Check sheet for the modelled part. Datum: model origin and axes. Units: mm. Face numbers are marked on the shaded views. A direction names the side the tool comes from. Round coordinates to 2 decimals unless told otherwise and drop trailing zeros. Write each loop counter-clockwise with the first axis right and the second up, starting at its lowest first coordinate (ties: lowest second). Pieces come first, ordered by that corner, then holes. Notation, with made-up numbers: (-34, 85) -> (7, 85) arc R24 cw to (7, 105) -> close; hole circle Ø8 at (67, -0.5). An arc over 180 degrees is marked (long way). One line per item, written item: value.
from build123d import *

# Parameters (mm, degrees)
SKETCH1_R           = 33.5
SKETCH1_R_2         = 30
BOSS_EXTRUDE1_DEPTH = 76.5
SKETCH3_R           = 33.5
BOSS_EXTRUDE2_DEPTH = 16.5
SKETCH4_W           = 20
SKETCH4_H           = 3.5
BOSS_EXTRUDE4_DEPTH = 30.867
SKETCH4_5_W         = 11
SKETCH4_5_H         = 3.5
BOSS_EXTRUDE5_DEPTH = 27
SKETCH4_7_R         = 1.25
CUT_EXTRUDE1_DEPTH  = 90.981942633
FILLET1_R           = 3.5
FILLET2_R           = 1.5
CUT_EXTRUDE4_DEPTH  = 103.136868955
BOSS_EXTRUDE7_START = 3
SKETCH6_10_R        = 10
BOSS_EXTRUDE7_DEPTH = 3
SKETCH12_R          = 5
SKETCH12_R_2        = 3
BOSS_EXTRUDE8_DEPTH = 1.5
SKETCH12_3_R        = 1.5
CUT_EXTRUDE7_DEPTH  = 101.439733174
CIRPATTERN1_COUNT   = 4
SKETCH12_4_R        = 1.5
CUT_EXTRUDE8_DEPTH  = 101.439733174
CUT_EXTRUDE9_DEPTH  = 90.981942633
CIRPATTERN2_COUNT   = 4
SKETCH13_W          = 60
SKETCH13_H          = 27
CUT_EXTRUDE11_DEPTH = 33.5
BOSS_EXTRUDE9_START = -3.5
SKETCH14_R          = 33.5
BOSS_EXTRUDE9_DEPTH = 3.5
CUT_EXTRUDE12_START = -4
CUT_EXTRUDE12_DEPTH = 4
CIRPATTERN3_COUNT   = 4
SKETCH16_R          = 2.7
CUT_EXTRUDE13_DEPTH = 10


with BuildPart() as part:
    # Sketch1 → Boss-Extrude1 (new body)
    with BuildSketch(Plane.XY):
        Circle(SKETCH1_R)
        Circle(SKETCH1_R_2, mode=Mode.SUBTRACT)
    extrude(amount=BOSS_EXTRUDE1_DEPTH)

    # Sketch3 → Boss-Extrude2 (add)
    with BuildSketch(Plane(origin=(0, 0, 0), x_dir=(-1, 0, 0), z_dir=(0, 0, -1))):
        with Locations(Location((0, 0, 0), (0, 0, 180))):
            Circle(SKETCH3_R)
    extrude(amount=-BOSS_EXTRUDE2_DEPTH)

    # Sketch4 → Boss-Extrude4 (add)
    with BuildSketch(Plane(origin=(0, 0, 0), x_dir=(-1, 0, 0), z_dir=(0, 0, -1))):
        with Locations((0, 27.05)):
            Rectangle(SKETCH4_W, SKETCH4_H)
    extrude(amount=BOSS_EXTRUDE4_DEPTH)

    # Sketch4_5 → Boss-Extrude5 (add)
    with BuildSketch(Plane(origin=(0, 0, 0), x_dir=(-1, 0, 0), z_dir=(0, 0, -1))):
        with Locations((0, -27.25)):
            Rectangle(SKETCH4_5_W, SKETCH4_5_H)
    extrude(amount=BOSS_EXTRUDE5_DEPTH)

    # Sketch4_7 → Cut-Extrude1 (cut, through all)
    with BuildSketch(Plane(origin=(0, 0, 0), x_dir=(-1, 0, 0), z_dir=(0, 0, -1))):
        Circle(SKETCH4_7_R)
    extrude(amount=-CUT_EXTRUDE1_DEPTH, mode=Mode.SUBTRACT)

    # Fillet1
    fillet1_edges = [part.edges().sort_by_distance(p)[0] for p in [
        (10, 27.05, 0),
        (-10, 27.05, 0),
    ]]
    fillet(fillet1_edges, radius=FILLET1_R)

    # Fillet2
    fillet2_edges = [part.edges().sort_by_distance(p)[0] for p in [
        (5.5, -27.25, 0),
        (-5.5, -27.25, 0),
    ]]
    fillet(fillet2_edges, radius=FILLET2_R)

    # Sketch6 → Cut-Extrude4 (cut, through all)
    with BuildSketch(Plane.XZ.offset(-25.3)):
        with BuildLine():
            Line((10, -30.867), (10, -20.77379065))
            ThreePointArc((10, -20.77379065), (0, -30.77379065), (-10, -20.77379065))
            Line((-10, -20.77379065), (-10, -30.867))
            Line((-10, -30.867), (10, -30.867))
        make_face()
    extrude(amount=-CUT_EXTRUDE4_DEPTH, mode=Mode.SUBTRACT)

    # Sketch6_10 → Boss-Extrude7 (add)
    with BuildSketch(Plane.XZ.offset(-25.3).offset(BOSS_EXTRUDE7_START)):
        with Locations(Location((0, -20.77379065, 0), (0, 0, 270))):
            Circle(SKETCH6_10_R)
    extrude(amount=-BOSS_EXTRUDE7_DEPTH)

    # Sketch12 → Boss-Extrude8 (add)
    with BuildSketch(Plane.XZ.offset(-22.3)):
        with Locations(Location((0, -20.77379065, 0), (0, 0, 270))):
            Circle(SKETCH12_R)
        with Locations(Location((0, -20.77379065, 0), (0, 0, 270))):
            Circle(SKETCH12_R_2, mode=Mode.SUBTRACT)
    extrude(amount=BOSS_EXTRUDE8_DEPTH)

    # Sketch12_3 → Cut-Extrude7 (cut, through all)
    with BuildSketch(Plane.XZ.offset(-22.3)):
        with Locations(Location((-7, -20.77379065, 0), (0, 0, 270))):
            Circle(SKETCH12_3_R)
    cut_extrude7 = extrude(amount=-CUT_EXTRUDE7_DEPTH, mode=Mode.SUBTRACT)

    # CirPattern1: Cut-Extrude7 ×4 about axis
    cirpattern1_axis = Axis((0, 0, -20.77379065), (0, 1, 0))
    for i in range(1, CIRPATTERN1_COUNT):
        add(cut_extrude7.rotate(cirpattern1_axis, i * 360 / CIRPATTERN1_COUNT), mode=Mode.SUBTRACT)

    # Sketch12_4 → Cut-Extrude8 (cut, through all)
    with BuildSketch(Plane.XZ.offset(-22.3)):
        with Locations(Location((0, -20.77379065, 0), (0, 0, 270))):
            Circle(SKETCH12_4_R)
    extrude(amount=-CUT_EXTRUDE8_DEPTH, mode=Mode.SUBTRACT)

    # Sketch4_8 → Cut-Extrude9 (cut, through all)
    with BuildSketch(Plane(origin=(0, 0, 0), x_dir=(-1, 0, 0), z_dir=(0, 0, -1))):
        with BuildLine():
            Line((15.588457268, 9), (7.794228634, 4.5))
            ThreePointArc((7.794228634, 4.5), (8.693332437, 2.329371406), (9, 0))
            Line((9, 0), (18, 0))
            ThreePointArc((18, 0), (17.386664873, 4.658742812), (15.588457268, 9))
        make_face()
        with BuildLine():
            ThreePointArc((9, 0), (8.693332437, -2.329371406), (7.794228634, -4.5))
            Line((7.794228634, -4.5), (15.588457268, -9))
            ThreePointArc((15.588457268, -9), (17.386664873, -4.658742812), (18, 0))
            Line((18, 0), (9, 0))
        make_face()
    cut_extrude9 = extrude(amount=-CUT_EXTRUDE9_DEPTH, mode=Mode.SUBTRACT)

    # CirPattern2: Cut-Extrude9 ×4 about axis
    cirpattern2_axis = Axis((0, 0, 0), (0, 0, -1))
    for i in range(1, CIRPATTERN2_COUNT):
        add(cut_extrude9.rotate(cirpattern2_axis, i * 360 / CIRPATTERN2_COUNT), mode=Mode.SUBTRACT)

    # Sketch13 → Cut-Extrude11 (cut)
    with BuildSketch(Plane(origin=(0, 33.5, 0), x_dir=(1, 0, 0), z_dir=(0, 1, 0))):
        with Locations((0, -38)):
            Rectangle(SKETCH13_W, SKETCH13_H)
    extrude(amount=-CUT_EXTRUDE11_DEPTH, mode=Mode.SUBTRACT)

    # Sketch14 → Boss-Extrude9 (add)
    with BuildSketch(Plane.XY.offset(76.5).offset(BOSS_EXTRUDE9_START)):
        Circle(SKETCH14_R)
    extrude(amount=BOSS_EXTRUDE9_DEPTH)

    # Sketch14_3 → Cut-Extrude12 (cut)
    with BuildSketch(Plane.XY.offset(76.5).offset(CUT_EXTRUDE12_START)):
        with BuildLine():
            Line((15.588457268, 9), (7.794228634, 4.5))
            ThreePointArc((7.794228634, 4.5), (8.693332437, 2.329371406), (9, 0))
            Line((9, 0), (18, 0))
            ThreePointArc((18, 0), (17.386664873, 4.658742812), (15.588457268, 9))
        make_face()
        with BuildLine():
            ThreePointArc((9, 0), (8.693332437, -2.329371406), (7.794228634, -4.5))
            Line((7.794228634, -4.5), (15.588457268, -9))
            ThreePointArc((15.588457268, -9), (17.386664873, -4.658742812), (18, 0))
            Line((18, 0), (9, 0))
        make_face()
    cut_extrude12 = extrude(amount=CUT_EXTRUDE12_DEPTH, mode=Mode.SUBTRACT)

    # CirPattern3: Cut-Extrude12 ×4 about axis
    cirpattern3_axis = Axis((0, 0, 16.5), (0, 0, -1))
    for i in range(1, CIRPATTERN3_COUNT):
        add(cut_extrude12.rotate(cirpattern3_axis, i * 360 / CIRPATTERN3_COUNT), mode=Mode.SUBTRACT)

    # Sketch16 → Cut-Extrude13 (cut)
    with BuildSketch(Plane.XZ.offset(29)):
        with BuildLine():
            Line((5.5, -27), (5.5, -20.77379065))
            ThreePointArc((5.5, -20.77379065), (0, -26.27379065), (-5.5, -20.77379065))
            Line((-5.5, -20.77379065), (-5.5, -27))
            Line((-5.5, -27), (5.5, -27))
        make_face()
        with Locations(Location((0, -20.77379065, 0), (0, 0, 270))):
            Circle(SKETCH16_R)
    extrude(amount=-CUT_EXTRUDE13_DEPTH, mode=Mode.SUBTRACT)


solid = part.part
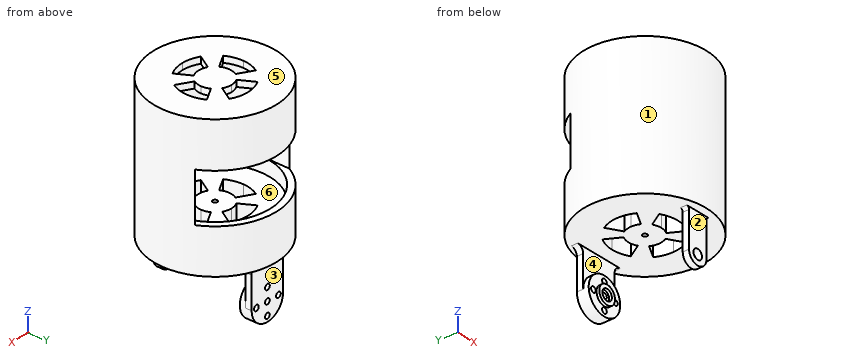
Item 1: Sectioned sample at A-A on y = 26.5. Enter the section's corners in (x, z).
Answer:
outline: (-20.49, 0) -> (-13.5, 0) arc R3.5 cw to (-10, -3.5) -> (-10, -20.77) arc R10 ccw to (10, -20.77) -> (10, -3.5) arc R3.5 cw to (13.5, 0) -> (20.49, 0) -> (20.49, 24.5) -> (14.06, 24.5) -> (14.06, 16.5) -> (-14.06, 16.5) -> (-14.06, 24.5) -> (-20.49, 24.5) -> close; (-20.49, 51.5) -> (-14.06, 51.5) -> (-14.06, 73) -> (14.06, 73) -> (14.06, 51.5) -> (20.49, 51.5) -> (20.49, 76.5) -> (-20.49, 76.5) -> close; hole circle Ø3 at (-7, -20.77); hole circle Ø3 at (0, -27.77); hole circle Ø3 at (0, -20.77); hole circle Ø3 at (0, -13.77); hole circle Ø3 at (7, -20.77)
Item 2: Tool access check on the marked faces 5 and 6. Record the directions out of +Z, -Z, +X, -X, +Y, -Y that give a thin tool (end or side, any length) a straight path to the whole face; none if there is none.
Answer:
face 5: +Z, +X, -X, +Y, -Y
face 6: none
Item 3: Sectioned sample at C-C on y = 19.5. Enter the section's corners in (x, z), and give its area (3 significant figures).
Answer:
outline: (-27.24, 0) -> (27.24, 0) -> (27.24, 24.5) -> (22.8, 24.5) -> (22.8, 16.5) -> (-22.8, 16.5) -> (-22.8, 24.5) -> (-27.24, 24.5) -> close; (-27.24, 51.5) -> (-22.8, 51.5) -> (-22.8, 73) -> (22.8, 73) -> (22.8, 51.5) -> (27.24, 51.5) -> (27.24, 76.5) -> (-27.24, 76.5) -> close
area: 1,350 mm^2
Item 4: Thickness scan on line 1 (Z direction, x = 8, y = 31); line 2 (Z direction, x = -25, y = -11); line 3 (Y direction, x = 0, z = 61). Record the ranges inside material, lowest first.
Answer:
line 1: z = 0 to 24.5, 51.5 to 76.5
line 2: z = 0 to 16.5, 73 to 76.5
line 3: y = -33.5 to -30, 30 to 33.5
Item 5: Sectioned sample at D-D on x = 25. Enter the section's corners in (y, z), and give its area (3 significant figures).
Answer:
outline: (-22.3, 0) -> (22.3, 0) -> (22.3, 24.5) -> (16.58, 24.5) -> (16.58, 16.5) -> (-16.58, 16.5) -> (-16.58, 73) -> (16.58, 73) -> (16.58, 51.5) -> (22.3, 51.5) -> (22.3, 76.5) -> (-22.3, 76.5) -> close
area: 1,380 mm^2
Item 6: Mould release check, pull along Y, two halves, no side actions. Record for the marked faces 1, 2, 3 and 4: pulls with the +Y half, pulls with the -Y half, needs draft (parallel to the pull), parting line crosses it, or undercut.
Answer:
face 1: parting line crosses it
face 2: pulls with the -Y half
face 3: pulls with the +Y half
face 4: undercut
Item 7: Depth check by flat-ended pin: P1, Ø16.5, axis at x = -1.5, z = -10, coming from the -Y side; P2, Ø3, axis at y = 27.5, z = -11.5, coming from the -X side; P3, Ø1.5, axis at y = -8.5, z = 38, coming from the -X side; P4, Ø6, axis at x = 12.5, y = -0.5, coming from the -Z side. Enter the tip coordinate at first touch or a pass-through.
Answer:
P1: stops at y = -29
P2: stops at x = -10
P3: stops at x = -32.59
P4: passes through
Item 8: Sectioned sample at B-B on z = 19. Enter the section's corners in (x, y).
Answer:
outline: circle Ø67 at (0, 0); hole circle Ø60 at (0, 0)
